```python
from build123d import *

# Parameters (mm, degrees)
BOSS_EXTRUDE1_DEPTH = 25
SKETCH2_W           = 400
SKETCH2_H           = 25
BOSS_EXTRUDE2_DEPTH = 150
CUT_EXTRUDE1_DEPTH  = 150
SKETCH4_R           = 7.94
CUT_EXTRUDE2_DEPTH  = 150
SKETCH5_R           = 20
CUT_EXTRUDE3_DEPTH  = 150


with BuildPart() as part:
    # Sketch1 → Boss-Extrude1 (new body)
    with BuildSketch(Plane.XY):
        with BuildLine():
            Line((-61.550518812, -258.970259643), (338.449481188, -258.970259643))
            Line((338.449481188, -258.970259643), (338.449481188, -148.970259643))
            ThreePointArc((338.449481188, -148.970259643), (326.733752435, -120.685988396), (298.449481188, -108.970259643))
            Line((298.449481188, -108.970259643), (236.429070899, -108.970259643))
            Line((236.429070899, -108.970259643), (136.429070899, -8.970259643))
            Line((136.429070899, -8.970259643), (136.429070899, 291.029740357))
            ThreePointArc((136.429070899, 291.029740357), (37.439276043, 376.851570008), (-61.550518812, 291.029740357))
            Line((-61.550518812, 291.029740357), (-61.550518812, -258.970259643))
        make_face()
    extrude(amount=BOSS_EXTRUDE1_DEPTH)

    # Sketch2 → Boss-Extrude2 (add)
    with BuildSketch(Plane.XY):
        with Locations((138.449481188, -246.470259643)):
            Rectangle(SKETCH2_W, SKETCH2_H)
    extrude(amount=BOSS_EXTRUDE2_DEPTH)

    # Sketch3 → Cut-Extrude1 (cut)
    with BuildSketch(Plane(origin=(0, -233.970259643, 0), x_dir=(1, 0, 0), z_dir=(0, 1, 0))):
        with BuildLine():
            Line((338.449481188, -110), (338.449481188, -150))
            Line((338.449481188, -150), (298.449481188, -150))
            ThreePointArc((298.449481188, -150), (326.733752435, -138.284271247), (338.449481188, -110))
        make_face()
        with BuildLine():
            Line((-61.550518812, -110), (-61.550518812, -150))
            Line((-61.550518812, -150), (-21.550518812, -150))
            ThreePointArc((-21.550518812, -150), (-49.83479006, -138.284271247), (-61.550518812, -110))
        make_face()
    extrude(amount=-CUT_EXTRUDE1_DEPTH, mode=Mode.SUBTRACT)

    # Sketch4 → Cut-Extrude2 (cut)
    with BuildSketch(Plane(origin=(0, -233.970259643, 0), x_dir=(1, 0, 0), z_dir=(0, 1, 0))):
        with Locations(Location((-21.550518812, -110, 0), (0, 0, 270))):
            Circle(SKETCH4_R)
        with Locations(Location((298.449481188, -110, 0), (0, 0, 270))):
            Circle(SKETCH4_R)
    extrude(amount=-CUT_EXTRUDE2_DEPTH, mode=Mode.SUBTRACT)

    # Sketch5 → Cut-Extrude3 (cut)
    with BuildSketch(Plane.XY.offset(25)):
        with Locations((37.439276043, 276.851570008)):
            Circle(SKETCH5_R)
        with Locations((58.449481188, -133.970259643)):
            Circle(SKETCH5_R)
    extrude(amount=-CUT_EXTRUDE3_DEPTH, mode=Mode.SUBTRACT)


solid = part.part
```
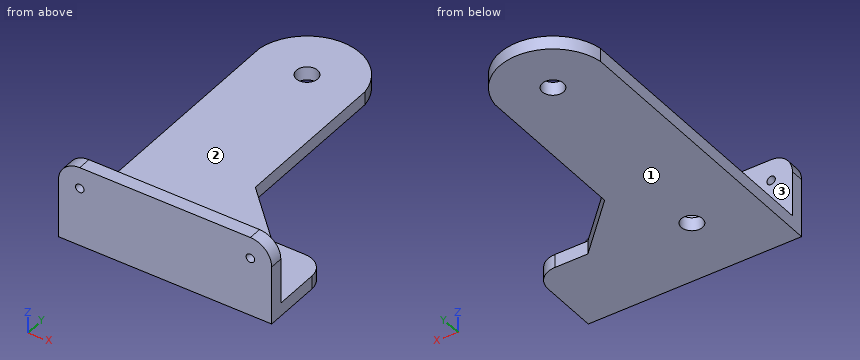
Geometry check sheet. Reference: the model listing, model coordinates, mm. Face numbers are marked on the shaded views. Coordinates: 2 decimals unless noted, no trailing zeros. Write each loop counter-clockwise with the first axis right and the second up, starting at its lowest first coordinate (ties: lowest second). Pieces come first, ordered by that corner, then holes. Notation, with made-up numbers: M 6,27 L 61,27 A26 ccw 61,65 Z; hole C 3,-28 d10. An arc over 180 degrees is marked long. One line per item, written item: value. Start each with the question number.
(1) Sectioned sample at B-B, the plane z = 126.5. Enter the section's corners in (x, y).
(2) Depth check by flat-ended pin: pin 1 (10 mm diameter, centred on y = 171, z = 25.5, fed in from +X); pin 2 (9.5 mm diameter, centred on x = 298.45, z = 110, fed in from -Y); pin 3 (6 mm diameter, centred on x = 115, y = -186.5, fed in from +Z); pin 4 (8 mm diameter, centred on x = 260, z = 57.5, fed in from +Y). Enter the tip coordinate at first touch or a pass-through.
(3) Scan lines: line 1 along X through (y, z) = (-247.5, 110); line 2 along Z through (x, y) = (93, 167); line 3 along Y through (x, z) = (212, 39). Record each from-to range of solid material in increasing order. Write a range as [from, to].
(4) Sectioned sample at A-A, the plane y = 209. Enter the section's corners in (x, z).
(5) Release check for a two-part mould opening along Z. For the marked faces 1, 2 and 3 record: released by +Z, released by -Z, zero draft, split by the parting line, or undercut.
Filled sheet:
1. outline: M -57.99,-258.97 L 334.89,-258.97 L 334.89,-233.97 L -57.99,-233.97 Z
2. pin 1: x = 136.43
2. pin 2: through
2. pin 3: z = 25
2. pin 4: y = -233.97
3. line 1: [-61.55, -29.49], [-13.61, 290.51], [306.39, 338.45]
3. line 2: [0, 25]
3. line 3: [-258.97, -233.97]
4. outline: M -61.55,0 L 136.43,0 L 136.43,25 L -61.55,25 Z
5. face 1: released by -Z
5. face 2: released by +Z
5. face 3: zero draft
